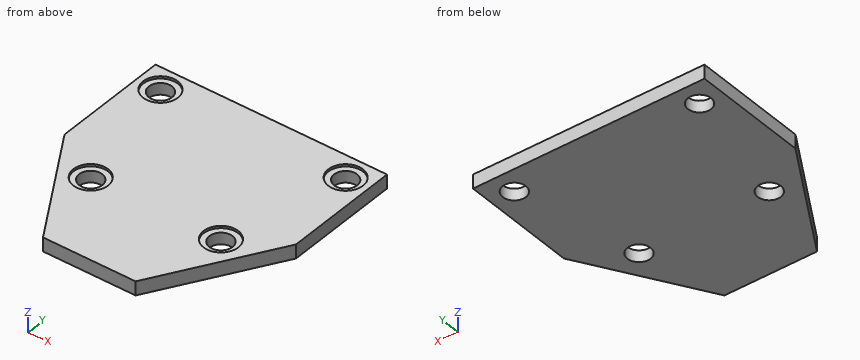
from build123d import *

# Parameters (mm, degrees)
F0_R     = 9.525
F2_DEPTH = 7.62
F0_R_2   = 6.35
F3_DEPTH = 6.35


with BuildPart() as f2:
    # F0 (on Top) → F2 (new body)
    with BuildSketch(Plane.XY):
        Polygon((-63.5, 0), (-25.4, -63.5), (25.4, -63.5), (63.5, 0), (63.5, 63.5), (-63.5, 63.5), align=None)
        with Locations((-35.722047, -17.059289)):
            Circle(F0_R, mode=Mode.SUBTRACT)
        with Locations((35.722047, -17.059289)):
            Circle(F0_R, mode=Mode.SUBTRACT)
        with Locations((-50.8, 50.8)):
            Circle(F0_R, mode=Mode.SUBTRACT)
        with Locations((50.8, 50.8)):
            Circle(F0_R, mode=Mode.SUBTRACT)
    extrude(amount=F2_DEPTH)

    # F0 (on Top) → F3 (join)
    with BuildSketch(Plane.XY):
        with Locations((-50.8, 50.8)):
            Circle(F0_R)
        with Locations((-50.8, 50.8)):
            Circle(F0_R_2, mode=Mode.SUBTRACT)
        with Locations((50.8, 50.8)):
            Circle(F0_R)
        with Locations((50.8, 50.8)):
            Circle(F0_R_2, mode=Mode.SUBTRACT)
        with Locations((35.722047, -17.059289)):
            Circle(F0_R)
        with Locations((35.722047, -17.059289)):
            Circle(F0_R_2, mode=Mode.SUBTRACT)
        with Locations((-35.722047, -17.059289)):
            Circle(F0_R)
        with Locations((-35.722047, -17.059289)):
            Circle(F0_R_2, mode=Mode.SUBTRACT)
    extrude(amount=F3_DEPTH)


solid = f2.part
Can you work these out from the model? Positions are in its coordinate system, mm. Round coordinates to 2 decimals unless told otherwise and drop trailing zeros. Write each loop counter-clockwise with the first axis right and the second up, starting at its lowest first coordinate (ties: lowest second). Pieces come first, ordered by that corner, then holes. Notation, with made-up numbers: (-37, -34.5) -> (14, -34.5) arc R29 ccw to (14, -0.5) -> close; hole circle Ø10 at (29, -1.75). An arc over 180 degrees is marked (long way). One line per question, with ' | ' between items. Start each with the question number.
1) Suppose I cut it at A-A on y = 50.8. Write out the boundary of the cut face in (x, z) (3 decimals), then the cut area to 3 significant figures.
2) Suppose I cut it at D-D on y = -51.5. Write out the boundary of the cut face in (x, z).
3) I need wall thicknesses on line 1 (X direction, y = -21.5, z = 1.25); line 2 (X direction, y = 52, z = 6); line 3 (Y direction, x = -50.8, z = 4.5). Which ranges of each line are inside material? Lowest first, please. Write a range as [from, to].
4) I'm going to push flat-ended pins straight in: P1, Ø2, axis at y = -46, z = 6.5, coming from the +X side; P2, Ø11.5, axis at x = -50.8, y = 50.8, coming from the -Z side; P3, Ø9.5, axis at x = -36, y = -14, coming from the +Z side. Where does each tip first touch, or does it pass through?
5) Suppose I cut it at B-B on z = 4.5. Write out the boundary of the cut face in (x, y).
6) Suppose I cut it at C-C on x = 53. Write out the boundary of the cut face in (y, z).
Return value:
1) outline: (-63.5, 0) -> (-57.15, 0) -> (-57.15, 6.35) -> (-60.325, 6.35) -> (-60.325, 7.62) -> (-63.5, 7.62) -> close; (-44.45, 0) -> (44.45, 0) -> (44.45, 6.35) -> (41.275, 6.35) -> (41.275, 7.62) -> (-41.275, 7.62) -> (-41.275, 6.35) -> (-44.45, 6.35) -> close; (57.15, 0) -> (63.5, 0) -> (63.5, 7.62) -> (60.325, 7.62) -> (60.325, 6.35) -> (57.15, 6.35) -> close | area: 758 mm2
2) outline: (-32.6, 0) -> (32.6, 0) -> (32.6, 7.62) -> (-32.6, 7.62) -> close
3) line 1: x = [-50.6, -40.26], [-31.18, 31.18], [40.26, 50.6] | line 2: x = [-63.5, -57.04], [-44.56, 44.56], [57.04, 63.5] | line 3: y = [-21.17, 44.45], [57.15, 63.5]
4) P1: stops at x = 36.5 | P2: passes through | P3: stops at z = 6.35
5) outline: (-63.5, 0) -> (-25.4, -63.5) -> (25.4, -63.5) -> (63.5, 0) -> (63.5, 63.5) -> (-63.5, 63.5) -> close; hole circle Ø12.7 at (-50.8, 50.8); hole circle Ø12.7 at (-35.72, -17.06); hole circle Ø12.7 at (35.72, -17.06); hole circle Ø12.7 at (50.8, 50.8)
6) outline: (-17.5, 0) -> (44.84, 0) -> (44.84, 6.35) -> (41.53, 6.35) -> (41.53, 7.62) -> (-17.5, 7.62) -> close; (56.76, 0) -> (63.5, 0) -> (63.5, 7.62) -> (60.07, 7.62) -> (60.07, 6.35) -> (56.76, 6.35) -> close
